Check sheet for the drawn part. Datum: minimum x, y, z corner. Units: mm. Coordinates: 2 decimals unless noted, no trailing zeros. Write each loop counter-clockwise with the first axis right and the second up, starting at its lowest first coordinate (ties: lowest second). Pieces come first, ordered by that corner, then holes. Notation, with made-up numbers: M -39,20.25 L 15,20.25 A7 ccw 15,26.25 Z; hole C 23,83.5 d1. An arc over 180 degrees is marked long. Answer as a JSON object with one key per item and string values. Group by question number.
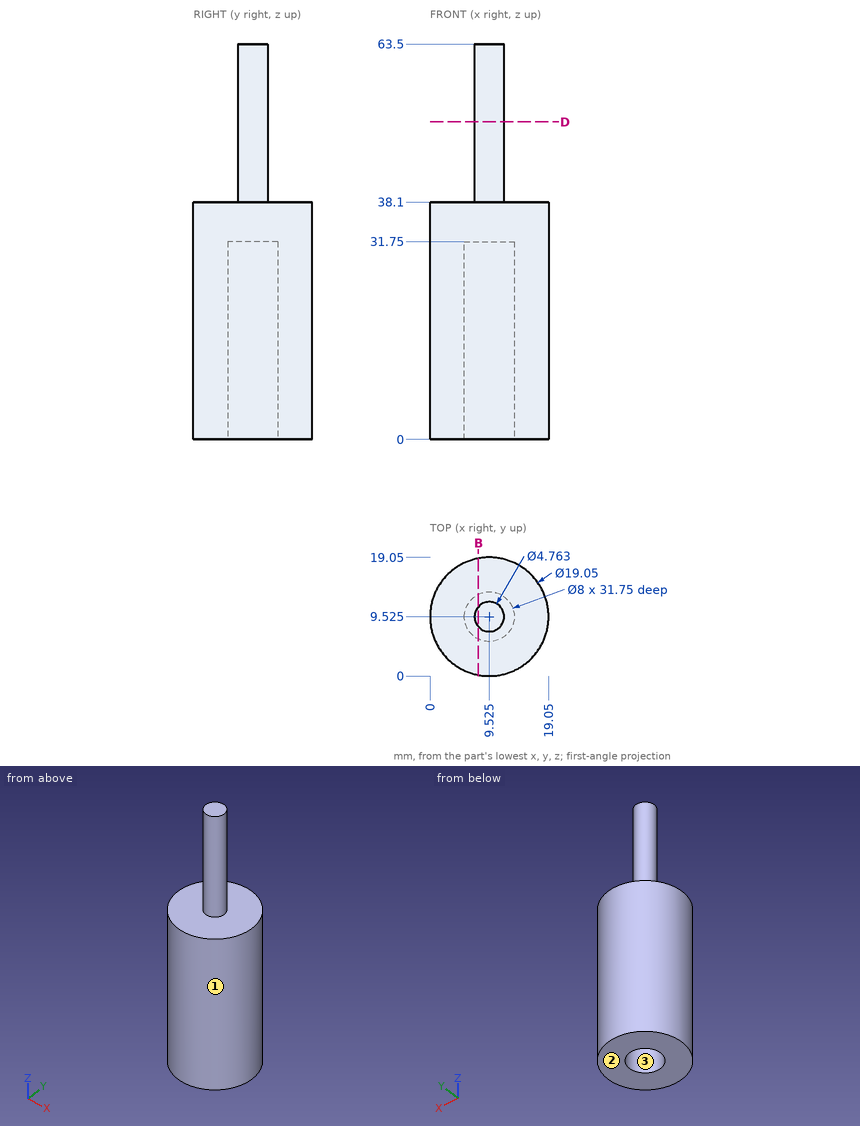
1) Section check B-B (x = 7.75). Record the cut outline in (y, z).
2) Section check D-D (z = 51). Record the cut outline in (x, y) (1 decimal), then the cut area to 3 significant figures.
3) Draft check along X on the marked faces 1, 2 and 3. Enter one of: +X half, -X half, draft (parallel to the pull), parting line (faces both ways), or undercut.
4) Go/stop test with flat-tipped pins: pin 1 Ø2.5 at (x, y) = (10, 10) entering from -Z; pin 2 Ø1 at (x, z) = (10, 44) entering from +Y; pin 3 Ø6 at (x, z) = (14.5, 11) entering from +Y. Record where each tip stops, or that it passes through.
5) Material ranges on probe 1 along Z at (x, y) = (3.75, 9.75); probe 2 along Z at (x, y) = (7.25, 6.5); probe 3 along X at (y, z) = (8, 9), recorded low to high. Write a range as [from, to].
Entries:
{
 "1": {"outline": "M 0.17,0 L 5.94,0 L 5.94,31.75 L 13.11,31.75 L 13.11,0 L 18.88,0 L 18.88,38.1 L 11.11,38.1 L 11.11,63.5 L 7.94,63.5 L 7.94,38.1 L 0.17,38.1 Z"},
 "2": {"outline": "C 9.5,9.5 d4.8", "area": "17.8 mm^2"},
 "3": {"face 1": "parting line", "face 2": "draft", "face 3": "undercut"},
 "4": {"pin 1": "z = 31.75", "pin 2": "y = 11.91", "pin 3": "y = 18.84"},
 "5": {"probe 1": "[0, 38.1]", "probe 2": "[31.75, 38.1]", "probe 3": "[0.12, 5.83], [13.22, 18.93]"}
}
